Read the model definition and answer for the solid it produces. Units are mm, in the model's axes. A direction names the side the tool comes from. Coordinates: 2 decimals unless noted, no trailing zeros. Loops run counter-clockwise (first coordinate to the right, second up) from the corner with the lowest first, then second, coordinate; pieces in that order, holes last.
Q1. Section C-C (z = -347.5) is taken. Give the vertices of the cut face in (x, y).
Q2. Straight lines are drawn through the part: line 1 (Y direction, x = 137, z = -170); line 2 (Z direction, x = 226, y = 21); line 3 (Z direction, x = 303.5, y = 15.5). For each, find the intervals that lie inside material, in ascending order.
Q3. Section A-A (x = 288) is taken. Give the vertices of the cut face in (y, z), then the cut area to 3 significant figures.
Q4. Flat-ended cylindrical pins translate along their axes: P1, Ø4, axis at x = 312, y = 27.5, coming from the +Z side; P2, Ø6, axis at x = 219.5, y = 11.5, coming from the -Z side. Find the tip coordinate at first contact, or state that the pin passes through.
Q5. Which of the six approach directions +Z, -Z, +X, -X, +Y, -Y give full straight-line access (tool end or side, diameter ignored) to faces 1 (the face through (400, 6, -172)), 2 (the face through (364.932, 20.638, 29.86)), 3 (the face through (45, 36, 20)), 4 (the face through (0, 6, -168)), 5 (the face through (44.97, 12.33, -369.86))?
Q6. Section D-D (x = 48) is taken. Give the vertices of the cut face in (y, z).
Q7. Section B-B (z = -168) is taken. Give the vertices of the cut face in (x, y).
Q8. The mould has two halves that part along Y. Classify faces 6 (the face through (364.932, 20.638, -369.86)), 7 (the face through (197.2, 20.53, -181.99)), 8 (the face through (385, 20, -15)): pulls with the +Y half, pulls with the -Y half, needs draft (parallel to the pull), parting line crosses it, or undercut.
from build123d import *

# Parameters (mm, degrees)
BOSS_EXTRUDE1_DEPTH = 40
SKETCH2_R           = 12
CUT_EXTRUDE1_DEPTH  = 401
SKETCH3_R           = 10
BOSS_EXTRUDE2_DEPTH = 20
SKETCH4_R           = 14
BOSS_EXTRUDE3_DEPTH = 20


with BuildPart() as part:
    # Sketch1 → Boss-Extrude1 (new body)
    with BuildSketch(Plane(origin=(0, 0, 0), x_dir=(1, 0, 0), z_dir=(0, 1, 0))):
        Polygon((0, 310), (30, 340), (370, 340), (400, 310), (400, 30), (370, 0), (30, 0), (0, 30), align=None)
    extrude(amount=BOSS_EXTRUDE1_DEPTH)

    # Sketch2 → Cut-Extrude1 (cut, through all)
    with BuildSketch(Plane.ZY):
        with Locations((-170, 20)):
            Circle(SKETCH2_R)
    extrude(amount=-CUT_EXTRUDE1_DEPTH, mode=Mode.SUBTRACT)

    # Sketch3 → Boss-Extrude2 (add)
    with BuildSketch(Plane.XY):
        with Locations((48, 26)):
            Circle(SKETCH3_R)
        with Locations((352, 26)):
            Circle(SKETCH3_R)
    boss_extrude2 = extrude(amount=BOSS_EXTRUDE2_DEPTH)

    # Sketch4 → Boss-Extrude3 (add)
    with BuildSketch(Plane.XY.offset(20)):
        with Locations((48, 26)):
            Circle(SKETCH4_R)
        with Locations((352, 26)):
            Circle(SKETCH4_R)
    boss_extrude3 = extrude(amount=BOSS_EXTRUDE3_DEPTH)

    # Mirror1: Boss-Extrude2, Boss-Extrude3 across plane
    add(boss_extrude2.mirror(Plane.XY.offset(-170)))
    add(boss_extrude3.mirror(Plane.XY.offset(-170)))


solid = part.part
Numbers:
1. outline: circle Ø20 at (48, 26); circle Ø20 at (352, 26)
2. line 1: y = 0 to 8, 32 to 40
2. line 2: z = -340 to -181.96, -158.04 to 0
2. line 3: z = -340 to -181.12, -158.88 to 0
3. outline: (0, -340) - (40, -340) - (40, 0) - (0, 0) - close; hole circle Ø24 at (20, -170)
3. area: 13,100 mm2
4. P1: stops at z = 0
4. P2: stops at z = -340
5. face 1: +Z, -Z, +X, +Y, -Y
5. face 2: +Z
5. face 3: none
5. face 4: +Z, -Z, -X, +Y, -Y
5. face 5: -Z
6. outline: (0, -340) - (16, -340) - (16, -360) - (12, -360) - (12, -380) - (40, -380) - (40, -360) - (36, -360) - (36, -340) - (40, -340) - (40, 0) - (36, 0) - (36, 20) - (40, 20) - (40, 40) - (12, 40) - (12, 20) - (16, 20) - (16, 0) - (0, 0) - close; hole circle Ø24 at (20, -170)
7. outline: (0, 0) - (400, 0) - (400, 8.17) - (0, 8.17) - close; (0, 31.83) - (400, 31.83) - (400, 40) - (0, 40) - close
8. face 6: parting line crosses it
8. face 7: undercut
8. face 8: needs draft
